Model file for the job. Use its own axes, mm. Round coordinates to 2 decimals unless told otherwise and drop trailing zeros. Loops run counter-clockwise (first coordinate to the right, second up) from the corner with the lowest first, then second, coordinate; pieces in that order, holes last. Notation, with made-up numbers: (-8, 11.25) - (47, 11.25) arc R24 ccw to (47, 36.25) - close; hole circle Ø9 at (84, 88.25). An arc over 180 degrees is marked (long way). Use one line per item in the form item = value.
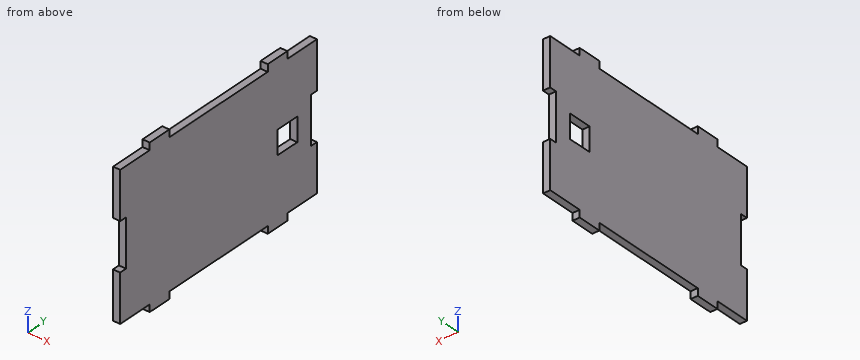
from build123d import *

# Parameters (mm, degrees)
SKETCH1_W           = 60
SKETCH1_H           = 100
BOSS_EXTRUDE1_DEPTH = 3
SKETCH2_W           = 3
SKETCH2_H           = 10
BOSS_EXTRUDE2_DEPTH = 3
SKETCH3_W           = 20
SKETCH3_H           = 3
CUT_EXTRUDE1_DEPTH  = 3
SKETCH4_W           = 10
SKETCH4_H           = 10
CUT_EXTRUDE2_DEPTH  = 3


with BuildPart() as part:
    # Sketch1 → Boss-Extrude1 (new body)
    with BuildSketch(Plane(origin=(0, 0, 0), x_dir=(0, 0, -1), z_dir=(1, 0, 0))):
        Rectangle(SKETCH1_W, SKETCH1_H)
    extrude(amount=BOSS_EXTRUDE1_DEPTH)

    # Sketch2 → Boss-Extrude2 (add)
    with BuildSketch(Plane(origin=(0, 0, 0), x_dir=(0, 0, -1), z_dir=(1, 0, 0))):
        with Locations((-31.5, -30)):
            Rectangle(SKETCH2_W, SKETCH2_H)
        with Locations((-31.5, 30)):
            Rectangle(SKETCH2_W, SKETCH2_H)
        with Locations((31.5, 30)):
            Rectangle(SKETCH2_W, SKETCH2_H)
        with Locations((31.5, -30)):
            Rectangle(SKETCH2_W, SKETCH2_H)
    extrude(amount=BOSS_EXTRUDE2_DEPTH)

    # Sketch3 → Cut-Extrude1 (cut)
    with BuildSketch(Plane(origin=(3, 0, 0), x_dir=(0, 0, -1), z_dir=(1, 0, 0))):
        with Locations((0, 48.5)):
            Rectangle(SKETCH3_W, SKETCH3_H)
        with Locations((0, -48.5)):
            Rectangle(SKETCH3_W, SKETCH3_H)
    extrude(amount=-CUT_EXTRUDE1_DEPTH, mode=Mode.SUBTRACT)

    # Sketch4 → Cut-Extrude2 (cut)
    with BuildSketch(Plane(origin=(3, 0, 0), x_dir=(0, 0, -1), z_dir=(1, 0, 0))):
        with Locations((0, 35)):
            Rectangle(SKETCH4_W, SKETCH4_H)
    extrude(amount=-CUT_EXTRUDE2_DEPTH, mode=Mode.SUBTRACT)


solid = part.part
1. Cut at A-A, the plane z = 3. Give the cut face in (x, y), plus the area to 3 significant figures.
Geometry check:
outline = (0, -47) - (3, -47) - (3, 30) - (0, 30) - close; (0, 40) - (3, 40) - (3, 47) - (0, 47) - close
area = 252 mm^2
2. Wall check: probe 1 along Y at (x, z) = (2.85, 30.5); probe 2 along Z at (x, y) = (2.6, 30.5); probe 3 along Z at (x, y) = (1, -17). Give the ranges that are in metal, low to high.
Geometry check:
probe_1 = -35 to -25, 25 to 35
probe_2 = -33 to -5, 5 to 33
probe_3 = -30 to 30
3. Cut at C-C, the plane y = 23.5. Give the cut face in (x, z), plus the area to 3 significant figures.
Geometry check:
outline = (0, -30) - (3, -30) - (3, 30) - (0, 30) - close
area = 180 mm^2
4. Flat gauge pins, fed straight in: pin 1 (1.5 mm diameter, centred on x = 1, y = -36, fed in from +Z); pin 2 (0.9 mm diameter, centred on x = 1.5, z = -31.5, fed in from -Y); pin 3 (0.9 mm diameter, centred on x = 1, z = -0.5, fed in from -Y). Where does each tip first touch, or does it go through?
Geometry check:
pin_1 = 30
pin_2 = -35
pin_3 = -47
